Source: three-view drawing plus pictorial views. Frame: mm from the lowest corner of the part. A direction names the side the tool comes from. Give positions to 0.01 mm unless a question says otherwise; leave off trailing zeros. Order: outer loops, then holes, each group sorted by start corner. A loop starts at its lowest first (then second) coordinate and runs counter-clockwise, first axis right, second up. Notation, with made-up numbers: M -14,60.5 L 42,60.5 A19 cw 42,80.5 Z; hole C -32.75,17.25 d10. An arc over 180 degrees is marked long. Use CSV: the item, a comma, the result in double quotes.
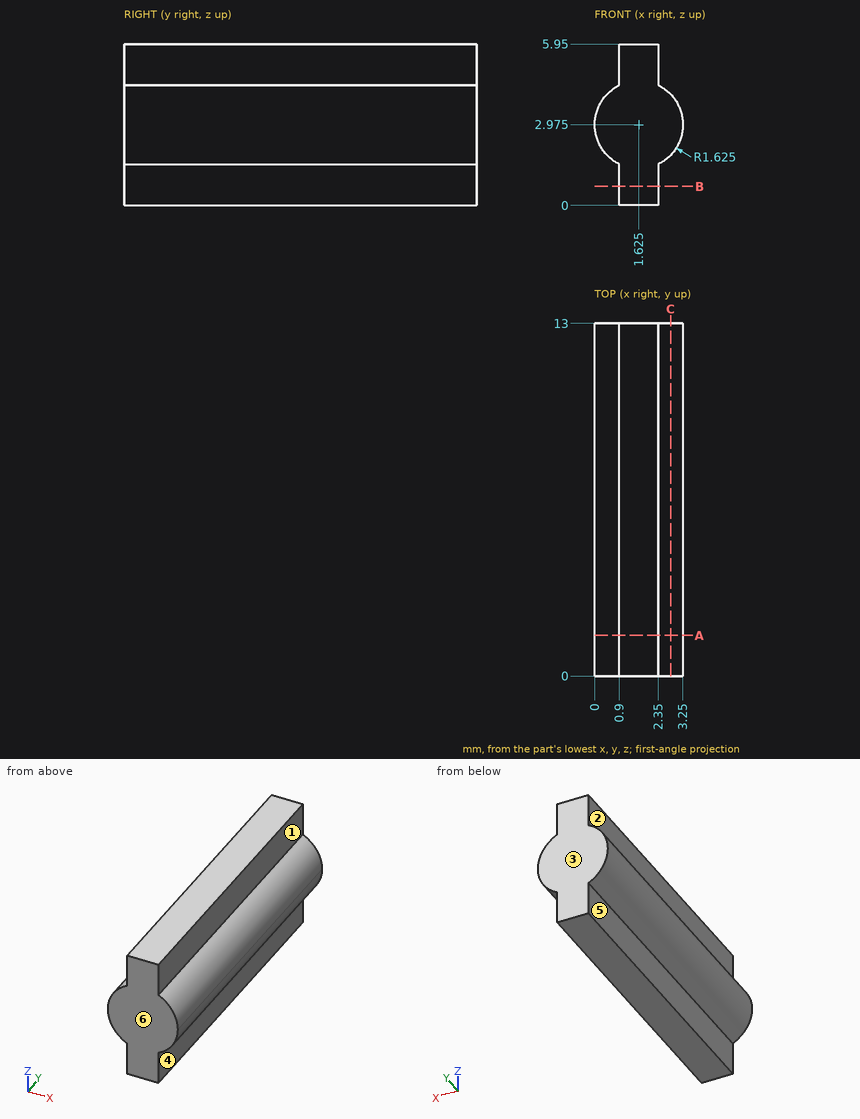
1. Pull-direction query (X, two-part tool) for the marked faces 1, 2 and 3; classes: +X half, -X half, draft (parallel to the pull), parting line (faces both ways), or undercut.
Answer:
face 1,"+X half"
face 2,"-X half"
face 3,"draft"
2. Reachability of the marked faces 4, 5 and 6 from +Z, -Z, +X, -X, +Y, -Y: full face, straight path, thin tool, end or side. Return the list, or none.
Answer:
face 4,"-Z, +X, +Y, -Y"
face 5,"-Z, -X, +Y, -Y"
face 6,"+Z, -Z, +X, -X, -Y"
3. Section C-C, the plane x = 2.8. Return the cut outline in (y, z).
Answer:
outline,"M 0,1.85 L 13,1.85 L 13,4.1 L 0,4.1 Z"
4. Pin query (flat end, axial travel): pin 1 Ø1.5 at (y, z) = (7.5, 4) entering from -X; pin 2 Ø0.5 at (y, z) = (4.5, 0.5) entering from -X; pin 3 Ø1.7 at (y, z) = (6, 5) entering from -X. Return the tip coordinate at first contact, or that it passes through.
Answer:
pin 1,"x = 0.02"
pin 2,"x = 0.9"
pin 3,"x = 0.5"
5. Section A-A, the plane y = 1.5. Return the cut outline in (x, z) (3 decimals), plus the area to 3 significant figures.
Answer:
outline,"M 0.9,0 L 2.35,0 L 2.35,1.521 A1.625 ccw 2.35,4.429 L 2.35,5.95 L 0.9,5.95 L 0.9,4.429 A1.625 ccw 0.9,1.521 Z"
area,"12.4 mm2"
6. Line query: line 1 (X direction, y = 10.5, z = 0.65); line 2 (Z direction, x = 3, y = 8.75); line 3 (Z direction, x = 2.6, y = 1.75) (3 decimals). Output: solid intervals per line, ascending.
Answer:
line 1,"0.9 to 2.35"
line 2,"2.11 to 3.84"
line 3,"1.675 to 4.275"
7. Section B-B, the plane z = 0.7. Return the cut outline in (x, y), plus the area to 4 significant figures.
Answer:
outline,"M 0.9,0 L 2.35,0 L 2.35,13 L 0.9,13 Z"
area,"18.85 mm2"
